Geometry: final body of the model. Coordinates: model frame, mm. A direction names the side the tool comes from. Coordinates: 2 decimals unless noted, no trailing zeros. Write each loop counter-clockwise with the first axis right and the second up, starting at its lowest first coordinate (ties: lowest second). Pieces come first, ordered by that corner, then holes. Notation, with made-up numbers: (73, 25) - (114, 25) arc R25 ccw to (114, 58) - close; hole circle Ø3 at (43.25, 72.25). An arc over 180 degrees is marked (long way). Answer as a JSON object with one key per item and string values. Group by question number.
Item 1: Set-up query: faces 4 (the flat face through (-30.5, 5, -11)), 5 (the cylindrical face through (-2.8, 4.9, -3.8)), 6 (the flat face through (-10, 2, -7.4)). Return all of +Z, -Z, +X, -X, +Y, -Y with unobstructed straight access to the full face (end or side cutting, diameter ignored); none if empty.
Item 2: Mould query, pull axis Y, two halves, no side actions, for faces 1 (the cylindrical face through (-25.2, 4.9, -17.7)), 2 (the flat face through (-10, 2.5, -4)), 3 (the flat face through (-19, 0, -7)). Classes: pulls with the +Y half, pulls with the -Y half, needs draft (parallel to the pull), parting line crosses it, or undercut.
Item 3: Section D-D on z = -5.5. Return loops of the section in (x, y), and give its area (3 significant figures).
Item 4: First-contact query: pin 1 Ø1 at (y, z) = (7.5, -8.5) entering from +X; pin 2 Ø6 at (x, y) = (-19.5, 5.5) entering from -Z. Flat tips, straight axial feed; report the tip coordinate or a pass-through.
Item 5: Section C-C on z = -2.75. Return loops of the section in (x, y).
Item 6: Line query: line 1 along Y through (x, z) = (-9.5, -4); line 2 along X through (y, z) = (5.25, -6); line 3 along X through (y, z) = (8.25, -13.25). Output: solid intervals per line, ascending. Write a range as from..to.
Item 7: Section A-A on y = 5. Return loops of the section in (x, z), and give its area (3 significant figures).
Item 8: Section B-B on x = -25.25. Return loops of the section in (y, z), and give its area (4 significant figures).
```python
from build123d import *

# Parameters (mm, degrees)
SKETCH1_R           = 2.55
BOSS_EXTRUDE1_DEPTH = 10
CUT_EXTRUDE1_DEPTH  = 34.709642537
FILLET2_R           = 1


with BuildPart() as part:
    # Sketch1 → Boss-Extrude1 (new body)
    with BuildSketch(Plane(origin=(0, 0, 0), x_dir=(1, 0, 0), z_dir=(0, 1, 0))):
        with BuildLine():
            Line((0, 0), (0, 7.4))
            Line((0, 7.4), (-20, 7.4))
            Line((-20, 7.4), (-20, 14.4))
            ThreePointArc((-20, 14.4), (-25.25, 17.7), (-30.5, 14.4))
            Line((-30.5, 14.4), (-30.5, 6.5))
            Line((-30.5, 6.5), (-24, 0))
            Line((-24, 0), (0, 0))
        make_face()
        with Locations(Location((-25.25, 11.873863636, 0), (0, 0, 270))):
            Circle(SKETCH1_R, mode=Mode.SUBTRACT)
    extrude(amount=BOSS_EXTRUDE1_DEPTH)

    # Sketch3 → Cut-Extrude1 (cut, through all)
    with BuildSketch(Plane(origin=(0, 0, -7.4), x_dir=(-1, 0, 0), z_dir=(0, 0, -1))):
        with BuildLine():
            Line((14, 2.5), (5.3, 2.5))
            ThreePointArc((5.3, 2.5), (2.8, 5), (5.3, 7.5))
            Line((5.3, 7.5), (14, 7.5))
            ThreePointArc((14, 7.5), (16.5, 5), (14, 2.5))
        make_face()
    extrude(amount=-CUT_EXTRUDE1_DEPTH, mode=Mode.SUBTRACT)

    # Fillet2
    fillet2_edges = [part.edges().sort_by_distance(p)[0] for p in [
        (-24, 5, 0),
        (-30.5, 5, -6.5),
        (-30.5, 5, -14.4),
        (-20, 5, -14.4),
        (-20, 5, -7.4),
        (0, 5, -7.4),
        (0, 5, 0),
    ]]
    fillet(fillet2_edges, radius=FILLET2_R)


solid = part.part
```
Checks:
{
 "1": {"face 4": "+Z, -Z, -X, +Y, -Y", "face 5": "+Z, -Z", "face 6": "-Z, +X, +Y, -Y"},
 "2": {"face 1": "needs draft", "face 2": "undercut", "face 3": "pulls with the -Y half"},
 "3": {"outline": "(-29.5, 0) - (0, 0) - (0, 10) - (-29.5, 10) - close; hole (-14, 2.5) - (-5.3, 2.5) arc R2.5 ccw to (-5.3, 7.5) - (-14, 7.5) arc R2.5 ccw to start", "area": "232 mm^2"},
 "4": {"pin 1": "x = -19.92", "pin 2": "z = -17.01"},
 "5": {"outline": "(-26.75, 0) - (0, 0) - (0, 10) - (-26.75, 10) - close; hole (-14, 2.5) - (-5.3, 2.5) arc R2.5 ccw to (-5.3, 7.5) - (-14, 7.5) arc R2.5 ccw to start"},
 "6": {"line 1": "0..2.5, 7.5..10", "line 2": "-30..-16.49, -2.81..0", "line 3": "-30.5..-27.4, -23.1..-20"},
 "7": {"outline": "(-30.5, -14.16) arc R1 ccw to (-30.38, -14.63) arc R5.83 ccw to (-20.12, -14.63) arc R1 ccw to (-20, -14.16) - (-20, -8.4) arc R1 cw to (-19, -7.4) - (-16.5, -7.4) - (-16.5, 0) - (-23.59, 0) arc R1 ccw to (-24.29, -0.29) - (-30.21, -6.21) arc R1 ccw to (-30.5, -6.91) - close; (-2.8, -7.4) - (-1, -7.4) arc R1 ccw to (0, -6.4) - (0, -1) arc R1 ccw to (-1, 0) - (-2.8, 0) - close; hole circle Ø5.1 at (-25.25, -11.87)", "area": "181 mm^2"},
 "8": {"outline": "(0, -17.7) - (10, -17.7) - (10, -14.42) - (0, -14.42) - close; (0, -9.32) - (10, -9.32) - (10, -1.25) - (0, -1.25) - close", "area": "113.5 mm^2"}
}
